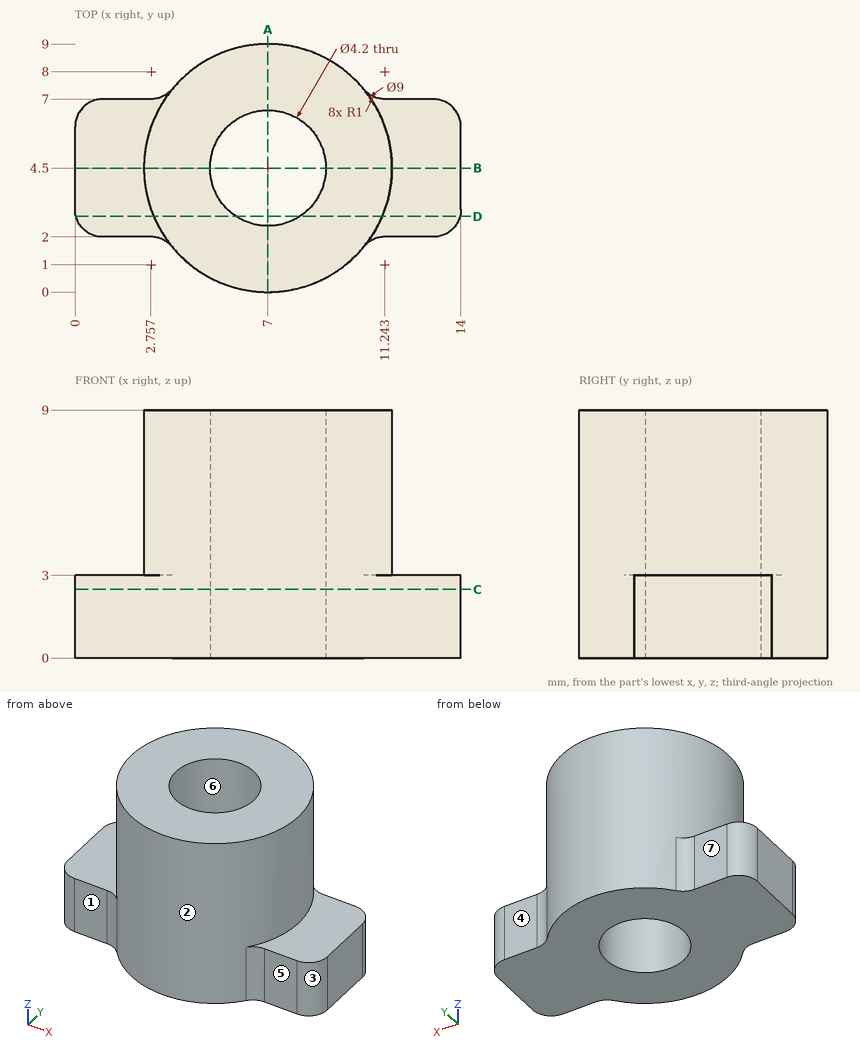
Study the drawing (mm; zero at the part's minimum x, y, z) and answer. A direction names the side the tool comes from. Coordinates: 2 decimals unless noted, no trailing zeros. Loops run counter-clockwise (first coordinate to the right, second up) from the corner with the lowest first, then second, coordinate; pieces in that order, holes last. Notation, with made-up numbers: M 22,88 L 29,88 A6 ccw 29,94 Z; hole C -14,55 d5. An arc over 180 degrees is marked long. Answer as a JSON object with one key per item and string values. Group by question number.
Item 1: Each of these flat-tipped pins is pushed along its axis until it touches: P1, Ø1.8, axis at x = 1, y = 3, coming from the +Z side; P2, Ø1.4, axis at x = 2, z = 2, coming from the +Y side; P3, Ø1.4, axis at x = 1.5, z = 1, coming from the -Y side. Where does it stop, or does it pass through?
Item 2: Determine the mould class of the marked faces 5, 6 and 7 for opening direction Y: +Y half, -Y half, draft (parallel to the pull), parting line (faces both ways), or undercut.
Item 3: Which of the six approach directions +Z, -Z, +X, -X, +Y, -Y give full straight-line access (tool end or side, diameter ignored) to the marked faces 1, 2, 3 and 4?
Item 4: Section D-D (y = 2.75) is taken. Write down the section's boundary in (x, z).
Item 5: Consider L1, parallel to Y at x = 7, z = 2; L2, parallel to Y at x = 6.5, z = 2; L3, parallel to Y at x = 12, z = 0.75. Determine where each line is inside the solid, lowest interval first.
Item 6: Section B-B (y = 4.5) is taken. Write down the section's boundary in (x, z), and give its area (3 significant figures).
Item 7: Section C-C (z = 2.5) is taken. Write down the section's boundary in (x, y).
Item 8: Section A-A (x = 7) is taken. Write down the section's boundary in (y, z).
Solved:
{
 "1": {"P1": "stops at z = 3", "P2": "stops at y = 7", "P3": "stops at y = 2"},
 "2": {"face 5": "-Y half", "face 6": "undercut", "face 7": "+Y half"},
 "3": {"face 1": "+Z, -Z, -X, -Y", "face 2": "+Z", "face 3": "+Z, -Z, +X, -Y", "face 4": "+Z, -Z, +X, +Y"},
 "4": {"outline": "M 0.03,0 L 5.84,0 L 5.84,9 L 2.85,9 L 2.85,3 L 0.03,3 Z; M 8.16,0 L 13.97,0 L 13.97,3 L 11.15,3 L 11.15,9 L 8.16,9 Z"},
 "5": {"L1": "y = 0 to 2.4, 6.6 to 9", "L2": "y = 0.03 to 2.46, 6.54 to 8.97", "L3": "y = 2 to 7"},
 "6": {"outline": "M 0,0 L 4.9,0 L 4.9,9 L 2.5,9 L 2.5,3 L 0,3 Z; M 9.1,0 L 14,0 L 14,3 L 11.5,3 L 11.5,9 L 9.1,9 Z", "area": "58.2 mm2"},
 "7": {"outline": "M 0,3 A1 ccw 1,2 L 2.76,2 A1 cw 3.53,1.64 A4.5 ccw 10.47,1.64 A1 cw 11.24,2 L 13,2 A1 ccw 14,3 L 14,6 A1 ccw 13,7 L 11.24,7 A1 cw 10.47,7.36 A4.5 ccw 3.53,7.36 A1 cw 2.76,7 L 1,7 A1 ccw 0,6 Z; hole C 7,4.5 d4.2"},
 "8": {"outline": "M 0,0 L 2.4,0 L 2.4,9 L 0,9 Z; M 6.6,0 L 9,0 L 9,9 L 6.6,9 Z"}
}
